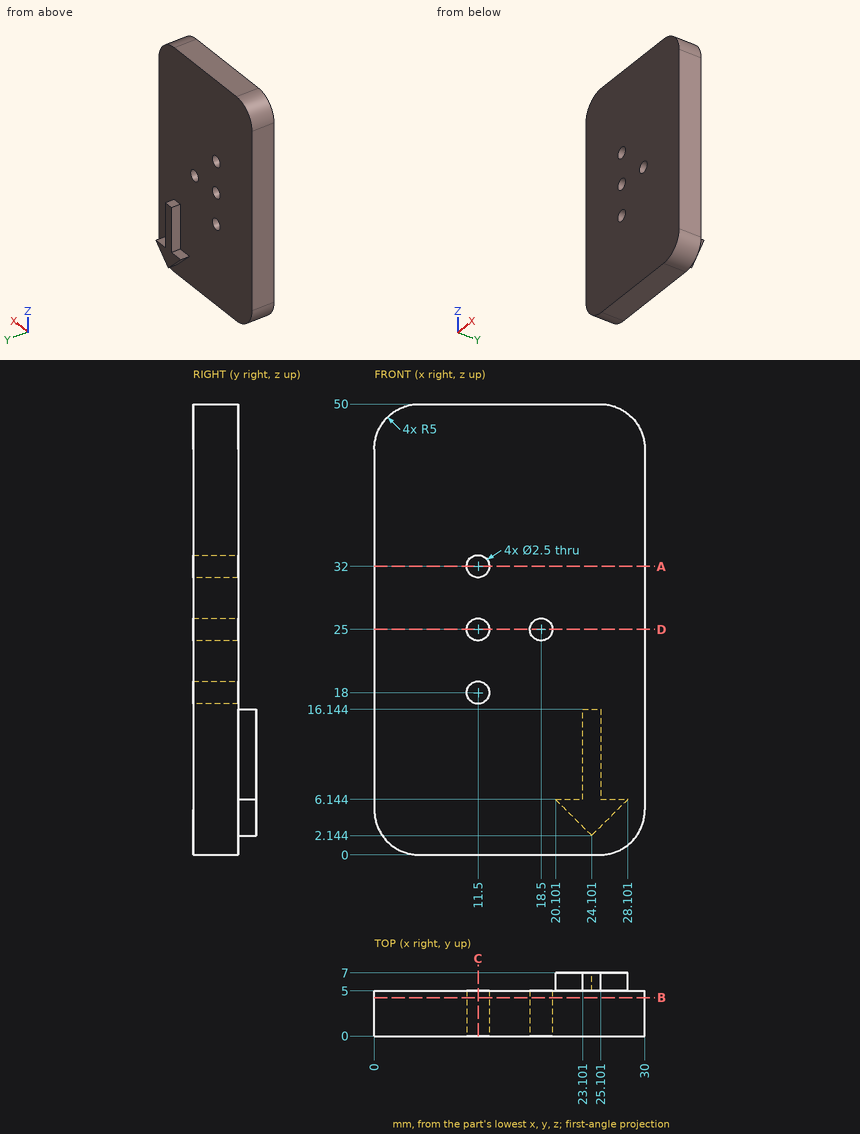
The drawing under review shows one solid part. Ordinate dimensions are in mm from its lowest x, y, z. Coordinates: 2 decimals unless noted, no trailing zeros. Order: outer loops, then holes, each group sorted by start corner. A loop starts at its lowest first (then second) coordinate and runs counter-clockwise, first axis right, second up. Notation, with made-up numbers: (31.25, -27.5) -> (89.25, -27.5) arc R12 ccw to (89.25, -11.5) -> close; hole circle Ø11 at (11.5, 68). An arc over 180 degrees is marked (long way). Answer as CSV lines item,"result".
Q1. We need section A-A (z = 32). State the section outline as (x, y) points, plus the area to 4 significant figures.
Model answer:
outline,"(0, 0) -> (10.25, 0) -> (10.25, 5) -> (0, 5) -> close; (12.75, 0) -> (30, 0) -> (30, 5) -> (12.75, 5) -> close"
area,"137.5 mm2"
Q2. We need section C-C (x = 11.5). State the section outline as (y, z) points.
Model answer:
outline,"(0, 0) -> (5, 0) -> (5, 16.75) -> (0, 16.75) -> close; (0, 19.25) -> (5, 19.25) -> (5, 23.75) -> (0, 23.75) -> close; (0, 26.25) -> (5, 26.25) -> (5, 30.75) -> (0, 30.75) -> close; (0, 33.25) -> (5, 33.25) -> (5, 50) -> (0, 50) -> close"
Q3. Clearance check with flat-ended pins moving along their axes: pin 1 Ø1.6 at (y, z) = (6, 10) entering from +X; pin 2 Ø9 at (x, z) = (15, 19.5) entering from +Y; pin 3 Ø2 at (x, y) = (24, 6.5) entering from +Z. State where each tip first meets the part, or that it passes through.
Model answer:
pin 1,"stops at x = 25.1"
pin 2,"stops at y = 5"
pin 3,"stops at z = 16.14"
Q4. We need section D-D (z = 25). State the section outline as (x, y) points, plus the area to 3 significant figures.
Model answer:
outline,"(0, 0) -> (10.25, 0) -> (10.25, 5) -> (0, 5) -> close; (12.75, 0) -> (17.25, 0) -> (17.25, 5) -> (12.75, 5) -> close; (19.75, 0) -> (30, 0) -> (30, 5) -> (19.75, 5) -> close"
area,"125 mm2"
Q5. Wall thickness on line 1 along X through (y, z) = (2.5, 25); line 2 along X through (y, z) = (4, 32); line 3 along Y through (x, z) = (13.5, 5): over which ranges is each line inside the solid? List them lowest first. Write a range as [from, to].
Model answer:
line 1,"x = [0, 10.25], [12.75, 17.25], [19.75, 30]"
line 2,"x = [0, 10.25], [12.75, 30]"
line 3,"y = [0, 5]"
Q6. We need section B-B (y = 4.25). State the section outline as (x, z) points.
Model answer:
outline,"(0, 5) arc R5 ccw to (5, 0) -> (25, 0) arc R5 ccw to (30, 5) -> (30, 45) arc R5 ccw to (25, 50) -> (5, 50) arc R5 ccw to (0, 45) -> close; hole circle Ø2.5 at (11.5, 18); hole circle Ø2.5 at (11.5, 25); hole circle Ø2.5 at (11.5, 32); hole circle Ø2.5 at (18.5, 25)"
